```python
from build123d import *

# Parameters (mm, degrees)
F0_R     = 1.5
F1_DEPTH = 5


with BuildPart() as f1:
    # F0 (on Front) → F1 (new body, symmetric)
    with BuildSketch(Plane.XZ):
        with BuildLine():
            Line((0, 2.5), (-138.000001, 2.5))
            ThreePointArc((-138.000001, 2.5), (-140.5, 0), (-138, -2.5))
            Line((-138, -2.5), (0, -2.5))
            ThreePointArc((0, -2.5), (2.5, 0), (0, 2.5))
        make_face()
        with Locations((-138, 0)):
            Circle(F0_R, mode=Mode.SUBTRACT)
        Circle(F0_R, mode=Mode.SUBTRACT)
    extrude(amount=F1_DEPTH, both=True)


solid = f1.part
```
Geometry check sheet. Reference: the model listing, model coordinates, mm. Round coordinates to 2 decimals unless told otherwise and drop trailing zeros. Order: outer loops, then holes, each group sorted by start corner. A loop starts at its lowest first (then second) coordinate and runs counter-clockwise, first axis right, second up. Notation, with made-up numbers: (8.25, 74) - (17.25, 74) arc R23 cw to (17.25, 87) - close; hole circle Ø2 at (-24.5, 40.25). An arc over 180 degrees is marked (long way). Use a Markdown table: item, result. Add a question column.
1) Thickness scan on line 1 along X through (y, z) = (-4.5, 0.1); line 2 along Z through (x, y) = (-138, 2.75); line 3 along X through (y, z) = (-3.5, 1.15). Record the ranges inside material, lowest first.
2) Section check B-B (y = 2.75). Record the cut outline in (x, z).
3) Section check A-A (z = 0). Record the cut outline in (x, y).
4) Gauge pin test, flat ends, axial feed: P1, Ø1.8, axis at x = 0, z = 0, coming from the -Y side; P2, Ø1.5, axis at y = -3.5, z = 1, coming from the -X side. Record the tip position at first contact, or that the pin passes through.
5) Mould release check, pull along Z, two halves, no side actions. Record for faces 1 (the cylindrical face through (2.5, -0.1, -0.1)), 2 (the cylindrical face through (-1.5, 0.07, 0.07)), 3 (the flat face through (-70, 0, -2.5)): released by +Z, released by -Z, zero draft, split by the parting line, or undercut.
Established:
| question | item | result |
|---|---|---|
| 1 | line 1 | -140.5 to -139.5, -136.5 to -1.5, 1.5 to 2.5 |
| 1 | line 2 | -2.5 to -1.5, 1.5 to 2.5 |
| 1 | line 3 | -140.22 to -138.96, -137.04 to -0.96, 0.96 to 2.22 |
| 2 | outline | (-138, -2.5) - (0, -2.5) arc R2.5 ccw to (0, 2.5) - (-138, 2.5) arc R2.5 ccw to start; hole circle Ø3 at (-138, 0); hole circle Ø3 at (0, 0) |
| 3 | outline | (-140.5, -5) - (-139.5, -5) - (-139.5, 5) - (-140.5, 5) - close; (-136.5, -5) - (-1.5, -5) - (-1.5, 5) - (-136.5, 5) - close; (1.5, -5) - (2.5, -5) - (2.5, 5) - (1.5, 5) - close |
| 4 | P1 | through |
| 4 | P2 | x = -140.49 |
| 5 | face 1 | split by the parting line |
| 5 | face 2 | undercut |
| 5 | face 3 | released by -Z |
